Could you check a few things on this drawing? It's one solid part, dimensions in mm from its lowest x, y, z. A direction names the side the tool comes from. Give positions to 0.01 mm unless a question says otherwise; leave off trailing zeros. Order: outer loops, then holes, each group sorted by start corner. A loop starts at its lowest first (then second) coordinate and runs counter-clockwise, first axis right, second up. Notation, with made-up numbers: (-13, 42.25) -> (-4, 42.25) arc R11 ccw to (-4, 47.25) -> close; hole circle Ø8 at (-38.75, -27). An arc over 180 degrees is marked (long way). Answer as a JSON object with one key per item and string values.
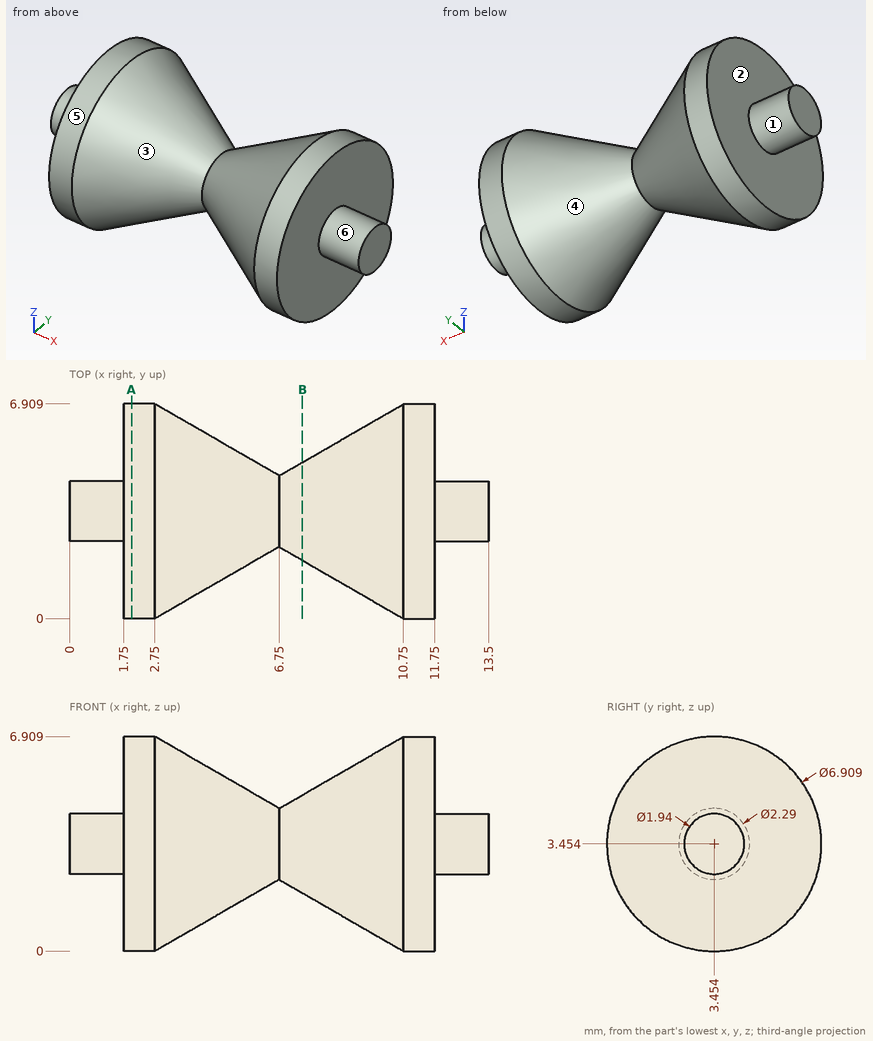
1. If we section it at A-A on x = 2: Please give me the cut outline in (y, z) (1 decimal), then the cut area to 3 significant figures.
Worked answers:
{"outline": "circle Ø6.9 at (3.5, 3.5)", "area": "37.5 mm²"}
2. For the marked faces 4, 5 and 6, which set-ups out of +Z, -Z, +X, -X, +Y, -Y let a thin tool reach every point of the face, with its end or its side?
Worked answers:
{"face 4": "none", "face 5": "+X, -X", "face 6": "+X"}
3. If we section it at B-B on x = 7.5: Please give me the cut outline in (y, z) (1 decimal).
Worked answers:
{"outline": "circle Ø3.2 at (3.5, 3.5)"}
4. If we mould it in two halves opening along X, with no side actions, what happens to the marked faces 1, 2 and 3? For each: +X half, -X half, draft (parallel to the pull), parting line (faces both ways), or undercut.
Worked answers:
{"face 1": "draft", "face 2": "-X half", "face 3": "undercut"}
5. Will this pin go through, and if not, where does the flat tip stop? pin 1 Ø1 at (x, y) = (9.5, 1) entering from +Z.
Worked answers:
{"pin 1": "z = 5.51"}
6. Please list where these lines run through material, in increasing order: L1, parallel to X at y = 3.5, z = 4.5; L2, parallel to X at y = 2.5, z = 2; L3, parallel to X at y = 3.5, z = 1.
Worked answers:
{"L1": "1.75 to 11.75", "L2": "1.75 to 5.72, 7.78 to 11.75", "L3": "1.75 to 4.48, 9.02 to 11.75"}
